Part model, mm, in its own coordinate system. A direction names the side the tool comes from. Coordinates: 2 decimals unless noted, no trailing zeros. Loops run counter-clockwise (first coordinate to the right, second up) from the corner with the lowest first, then second, coordinate; pieces in that order, holes last. Notation, with made-up numbers: M 2,74 L 21,74 A31 ccw 21,105 Z; hole C 60,-5.75 d2. An arc over 180 degrees is marked long. Use CSV: the item, a comma, the result in double quotes. Start each with the question number.
Autodesk Inventor part; units mm, degrees
ref_plane "YZ Plane" through (0, 0, 0) normal (1, 0, 0) x (0, 1, 0)
ref_plane "XZ Plane" through (0, 0, 0) normal (0, 1, 0) x (-1, 0, 0)
ref_plane "XY Plane" through (0, 0, 0) normal (0, 0, 1) x (1, 0, 0)
sketch "Sketch4" plane through (0, 0, 0) normal (0, 1, 0) x (-1, 0, 0)
  circle A0 centre (0, 0) radius 2.5
extrude "Extrusion2" add sketch "Sketch4" along normal mid plane 37
chamfer "Chamfer1" distance 0.5 angle 45 1 edges at (2.5, 18.5, 0)
sketch "Sketch14" plane through (0, -18.5, 0) normal (0, -1, 0) x (1, 0, 0)
  circle A0 centre (0, 0) radius 4
  dimension "d101" = 8
extrude "Extrusion10" add sketch "Sketch14" along normal blind 3
sketch "Sketch15" plane through (0, 0, 0) normal (0, 0, 1) x (1, 0, 0)
  line L0 (-2.5, -18.5) -> (-2.5, 18)
  line L1 (-2.5, -12.7) -> (-2, -12.7)
  line L2 (-2, -12.7) -> (-2, -13.5)
  line L3 (-2, -13.5) -> (-2.5, -13.5)
  line L4 (-2.5, -13.5) -> (-2.5, -12.7)
  line L5 (0, -22.5133) -> (0, 22.052) construction
  line L6 (-4, -18.5) -> (4, -18.5)
  point P0 (0, 0)
  dimension "d104" = 2
  dimension "d105" = 0.8
  dimension "d106" = 5
revolve "Revolution1" cut sketch "Sketch15" angle 360 about axis through (0, -22.5133, 0) along (0, 1, 0)
chamfer "Chamfer2" distance 0.1 angle 45 2 edges at (-4, -18.5, 0) (-4, -21.5, 0)
sketch "Sketch16" plane through (0, 0, 0) normal (1, 0, 0) x (0, 1, 0)
  line L0 (28.5, 0.5) -> (3.5, 0.5)
  line L1 (3.5, 0.5) -> (3.5, -0.5)
  line L2 (3.5, -0.5) -> (28.5, -0.5)
  line L3 (28.5, -0.5) -> (28.5, 0.5)
  line L4 (28.5, 0.5) -> (3.5, -0.5) construction
  line L5 (3.5, 0.5) -> (28.5, -0.5) construction
  line L6 (18.5, 2) -> (18.5, -2)
  point P0 (0, 0)
  point P1 (16, 0)
  dimension "d111" = 15
  dimension "d112" = 1
  dimension "d115" = 10
extrude "Extrusion11" cut sketch "Sketch16" against normal mid plane 7.75
properties part number "Wheel Handle" material "Bronze, Soft Tin"
1. Slice it at B-B, the plane y = 8. List the corners of the cut face in (x, z).
2. Slice it at A-A, the plane z = 0. List the corners of the cut face in (x, y).
3. Pin check, flat tips, straight feed: pin 1 (1 mm diameter, centred on x = -1.5, y = -4.5, fed in from -Z); pin 2 (2 mm diameter, centred on y = -14, z = 0, fed in from +X); pin 3 (2.5 mm diameter, centred on x = 0, y = 13.5, fed in from +Z). Stop position of each tip, or through.
4. Tool access for faces 1 (the face through (1, -12.7, 2)), 2 (the face through (0, 3.5, 0)), 3 (the face through (0, -18.5, -3)): list every direction of +Z, -Z, +X, -X, +Y, -Y with a clear straight run to the whole face (end or side of a thin tool).
5. Slice it at D-D, the plane y = -17. List the corners of the cut face in (x, z).
6. Two-plate mould, pull along Z, no slides. Class faces 4 (the face through (0, 11, 0.5)), 5 (the face through (-0.04, 18.36, -2.14)), 6 (the face through (0, 11, -0.5)), 7 (the face through (0.04, 18.36, 2.14)): pulls with the +Z half, pulls with the -Z half, needs draft (parallel to the pull), parting line crosses it, or undercut.
7. Slice it at C-C, the plane x = 0. List the corners of the cut face in (y, z), and give its area (3 significant figures).
8. Wall check: probe 1 along Y at (x, z) = (0.5, -2.5); probe 2 along Z at (x, y) = (-0.5, -3.5); probe 3 along Z at (x, y) = (-1.5, -1). Give the ranges that are in metal, low to high.
Found:
1,outline,"M -2.45,-0.5 A2.5 ccw 2.45,-0.5 Z; M -2.45,0.5 L 2.45,0.5 A2.5 ccw Z"
2,outline,"M -4,-21.4 L -3.9,-21.5 L 3.9,-21.5 L 4,-21.4 L 4,-18.6 L 3.9,-18.5 L 2.5,-18.5 L 2.5,-13.5 L 2,-13.5 L 2,-12.7 L 2.5,-12.7 L 2.5,3.5 L -2.5,3.5 L -2.5,-12.7 L -2,-12.7 L -2,-13.5 L -2.5,-13.5 L -2.5,-18.5 L -3.9,-18.5 L -4,-18.6 Z"
3,pin 1,"z = -2.29"
3,pin 2,"x = 2.5"
3,pin 3,"z = 2.5"
4,face 1,"none"
4,face 2,"+X, -X, +Y"
4,face 3,"+Y"
5,outline,"C 0,0 d5"
6,face 4,"undercut"
6,face 5,"pulls with the -Z half"
6,face 6,"undercut"
6,face 7,"pulls with the +Z half"
7,outline,"M -21.5,-3.9 L -21.4,-4 L -18.6,-4 L -18.5,-3.9 L -18.5,-2.5 L -13.5,-2.5 L -13.5,-2 L -12.7,-2 L -12.7,-2.5 L 18,-2.5 L 18.5,-2 L 18.5,-0.5 L 3.5,-0.5 L 3.5,0.5 L 18.5,0.5 L 18.5,2 L 18,2.5 L -12.7,2.5 L -12.7,2 L -13.5,2 L -13.5,2.5 L -18.5,2.5 L -18.5,3.9 L -18.6,4 L -21.4,4 L -21.5,3.9 Z"
7,area,"193 mm^2"
8,probe 1,"-21.5 to -18.5"
8,probe 2,"-2.45 to 2.45"
8,probe 3,"-2 to 2"
